Autodesk Fusion 360 part; units mm, degrees
sketch "Sketch Metalens Holder" plane through (0, 0, 0) normal (1, 0, 0) x (0, 0, -1)
  line L0 (0, 8.15) -> (16.5, 8.15)
  line L1 (16.5, 8.15) -> (16.5, -8.35)
  line L2 (16.5, -8.35) -> (0, -8.35)
  line L3 (0, -8.35) -> (0, 8.15)
  dimension "d3" = 16.5
  dimension "d4" = 16.5
extrude "Extrude Metalens Holder" add sketch "Sketch Metalens Holder" along normal blind 6
shell "Shell Metalens Holder" thickness 1.1 removed faces 2 at (6, 2.65, -5.5) at (0, 2.65, -5.5)
sketch "Sketch Screwing Parts" plane through (0, 0, 0) normal (1, 0, 0) x (0, 0, -1)
  line L0 (0, -8.35) -> (16.5, -8.35)
  line L1 (3.5, 8.15) -> (18, 8.15)
  line L2 (18, 8.15) -> (18, 35.85)
  line L3 (18, 35.85) -> (3.5, 35.85)
  line L4 (3.5, 35.85) -> (3.5, 8.15)
  line L5 (3.5, -8.35) -> (18, -8.35)
  line L6 (18, -8.35) -> (18, -36.05)
  line L7 (18, -36.05) -> (3.5, -36.05)
  line L8 (3.5, -36.05) -> (3.5, -8.35)
  line L9 (16.5, -8.35) -> (16.5, 8.15)
  point P0 (0, 8.15)
  dimension "d144" = 3.5
  dimension "d145" = 27.7
  dimension "d148" = 27.7
  dimension "d163" = 1.5
  dimension "d164" = 3.5
extrude "Extrude31" add sketch "Sketch Screwing Parts" along normal blind 6
ref_plane "WorkPlane1" through (3, -0.1, -8.25) normal (-1, 0, 0) x (0, 0, 1)
sketch "Sketch Inside Slit" plane through (3, 0, 0) normal (-1, 0, 0) x (0, 0, 1)
  line L0 (-15.4, 7.05) -> (-15.4, -7.25)
  line L1 (-16, 7.65) -> (-0.5, 7.65)
  line L2 (-0.5, 7.65) -> (-0.5, -7.85)
  line L3 (-0.5, -7.85) -> (-16, -7.85)
  line L4 (-16, -7.85) -> (-16, 7.65)
  line L5 (-15.4, 7.05) -> (-1.1, 7.05)
  line L6 (-1.1, 7.05) -> (-1.1, -7.25)
  line L7 (-1.1, -7.25) -> (-15.4, -7.25)
  line L8 (-15.4, -7.25) -> (-15.4, 7.05)
  line L9 (-15.4, 7.05) -> (-16, 7.05)
  line L10 (-1.1, 7.05) -> (-0.5, 7.05)
  line L11 (-1.1, -7.25) -> (-0.5, -7.25)
  line L12 (-15.4, -7.25) -> (-16, -7.25)
  point P0 (-1.1, -7.25)
  point P1 (-1.1, 7.05)
  dimension "d91" = 15.5
extrude "Extrude Inside Slit" cut sketch "Sketch Inside Slit" along normal mid plane 1 contours L2 L6 L10 L11
extrude "Extrude Inside Slit Bis" cut sketch "Sketch Inside Slit" along normal mid plane 1 contours L1 L2 L4 L5 L9 L10
extrude "Extrude Inside Slit BisBis" cut sketch "Sketch Inside Slit" along normal mid plane 1 contours L0 L4 L8 L9 L12
extrude "Extrude Inside Slit BisBisBis" cut sketch "Sketch Inside Slit" along normal mid plane 1
extrude "Extrude" cut 1 faces at (0.8333, 2.2833, -15.4) along direction (0, 0, -1) blind 1.1
extrude "Extrude22" cut 1 faces at (4.3333, 2.2833, -15.4) along direction (0, 0, -1) blind 1.1
extrude "Extrude23" cut 1 faces at (2.8333, -2.4833, -16) along direction (0, 0, -1) blind 0.5
extrude "Extrude24" add 1 faces at (2, -2.85, 0) along direction (0, 0, 1) blind 0.9
extrude "Extrude25" add 2 faces at (2, 8.15, -2.0333) (2, 8.15, -2.0333) along direction (0, 1, 0) blind 0.9
extrude "Extrude26" add 2 faces at (2, -8.35, -2.0333) (2, -8.35, -2.0333) along direction (0, -1, 0) blind 0.9
extrude "Extrude27" add 1 faces at (6, 26.9167, -8.3333) along direction (1, 0, 0) blind 4.5
extrude "Extrude28" add 1 faces at (0, 26.9167, -8.3333) along direction (-1, 0, 0) blind 4.5
extrude "Extrude29" add 1 faces at (-2.1667, 7.6167, -16.5) along direction (0, 0, -1) blind 1.5
extrude "Extrude30" add 1 faces at (-2.1667, -7.8167, -16.5) along direction (0, 0, -1) blind 1.5
sketch "Sketch11" plane through (0, 0, -18) normal (0, 0, -1) x (-1, 0, 0)
  line L0 (4.5, 35.85) -> (-10.5, 35.85)
  line L1 (-10.5, 35.85) -> (-10.5, 7.05)
  line L2 (-10.5, 7.05) -> (-3.5, 7.05)
  line L3 (-3.5, 7.05) -> (-3.5, 7.65)
  line L4 (-3.5, 7.65) -> (-2.5, 7.65)
  line L5 (-2.5, 7.65) -> (-2.5, 7.05)
  line L6 (4.5, 7.05) -> (4.5, 35.85)
  circle A0 centre (-3, 30.3) radius 3.75
  line L7 (-2.5, 7.05) -> (4.5, 7.05)
  dimension "d154" = 7.5
extrude "Extrude32" cut sketch "Sketch11" against normal blind 14.5 contours A0
sketch "Sketch12" plane through (0, 0, -18) normal (0, 0, -1) x (-1, 0, 0)
  line L0 (-10.5, -7.25) -> (-10.5, -36.05)
  line L1 (-10.5, -36.05) -> (4.5, -36.05)
  line L2 (4.5, -36.05) -> (4.5, -7.25)
  line L3 (4.5, -7.25) -> (-2.5, -7.25)
  line L4 (-2.5, -7.25) -> (-2.5, -7.85)
  line L5 (-2.5, -7.85) -> (-3.5, -7.85)
  line L6 (-3.5, -7.85) -> (-3.5, -7.25)
  line L7 (-3.5, -7.25) -> (-10.5, -7.25)
  circle A0 centre (-2.9472, -30.4996) radius 3.75
  dimension "d159" = 7.5
extrude "Extrude33" cut sketch "Sketch12" against normal blind 14.5 contours A0
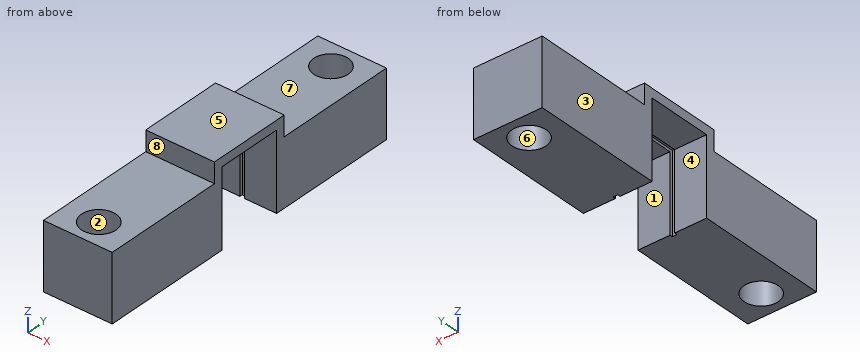
Work out the finished part from the listing and answer in its coordinate system (mm). Face numbers are marked on the shaded views. A direction names the side the tool comes from. Round coordinates to 2 decimals unless told otherwise and drop trailing zeros. Loops run counter-clockwise (first coordinate to the right, second up) from the corner with the lowest first, then second, coordinate; pieces in that order, holes last. Notation, with made-up numbers: (11, 37) - (38, 37) arc R27 ccw to (38, 73) - close; hole circle Ø4 at (59.5, 87). An arc over 180 degrees is marked (long way). Use one line per item in the form item = value. Start each with the question number.
(1) Find section A-A on z = -10.5. Determine the outline of the cut face in (x, y), and give its area (3 significant figures).
(2) Determine the mould class of the marked faces 1, 2 and 3 for opening direction X: +X half, -X half, draft (parallel to the pull), parting line (faces both ways), or undercut.
(3) Find section C-C on x = 1. Determine the outline of the cut face in (y, z), and give its area (3 significant figures).
(4) Find section B-B on y = 30.3. Determine the outline of the cut face in (x, z), and give its area (3 significant figures).
(5) Flat-ended cylindrical pins translate along their axes: P1, Ø8, axis at y = -3.5, z = -7, coming from the +X side; P2, Ø5.5, axis at x = 8, y = 1, coming from the -Z side; P3, Ø2, axis at x = 1, z = -0.5, coming from the -Y side; P4, Ø3.5, axis at x = 2, z = -0.5, coming from the +Y side. Find the tip coordinate at first contact, or state that the pin passes through.
(6) Which of the six approach directions +Z, -Z, +X, -X, +Y, -Y give full straight-line access (tool end or side, diameter ignored) to the marked faces 4, 5, 6, 7 and 8?
(7) Consider line 1 (Y direction, x = 3, z = -14.5); line 2 (Y direction, x = 1.5, z = -15.25); line 3 (Y direction, x = 4.75, z = -2.5). Determine where each line is inside the solid, lowest interval first.
(8) Find section D-D on y = 2.5. Determine the outline of the cut face in (x, z).
Answer list:
q1.outline = (-4.5, -36.05) - (10.5, -36.05) - (10.5, -7.25) - (3.5, -7.25) - (3.5, -7.85) - (2.5, -7.85) - (2.5, -7.25) - (-4.5, -7.25) - close; (-4.5, 7.05) - (2.5, 7.05) - (2.5, 7.65) - (3.5, 7.65) - (3.5, 7.05) - (10.5, 7.05) - (10.5, 35.85) - (-4.5, 35.85) - close; hole circle Ø7.5 at (2.95, -30.5); hole circle Ø7.5 at (3, 30.3)
q1.area = 774 mm^2
q2.face_1 = draft
q2.face_2 = undercut
q2.face_3 = -X half
q3.outline = (-36.05, -18) - (-33.7, -18) - (-33.7, -3.5) - (-36.05, -3.5) - close; (-27.29, -18) - (-7.25, -18) - (-7.25, -1.1) - (7.05, -1.1) - (7.05, -18) - (27.13, -18) - (27.13, -3.5) - (9.05, -3.5) - (9.05, 0.9) - (-9.25, 0.9) - (-9.25, -3.5) - (-27.29, -3.5) - close; (33.47, -18) - (35.85, -18) - (35.85, -3.5) - (33.47, -3.5) - close
q3.area = 696 mm^2
q4.outline = (-4.5, -18) - (-0.75, -18) - (-0.75, -3.5) - (-4.5, -3.5) - close; (6.75, -18) - (10.5, -18) - (10.5, -3.5) - (6.75, -3.5) - close
q4.area = 109 mm^2
q5.P1 = 10.5
q5.P2 = -1.1
q5.P3 = -9.25
q5.P4 = 9.05
q6.face_4 = -Z, +X, -X
q6.face_5 = +Z, +X, -X, +Y, -Y
q6.face_6 = +Z, -Z
q6.face_7 = +Z, +X, -X, +Y
q6.face_8 = +Z, +X, -X, -Y
q7.line_1 = -36.05 to -34.25, -26.75 to -7.85, 7.65 to 26.55, 34.05 to 35.85
q7.line_2 = -36.05 to -33.96, -27.04 to -7.25, 7.05 to 26.86, 33.74 to 35.85
q7.line_3 = -9.25 to -7.25, 7.05 to 9.05
q8.outline = (-4.5, -1.1) - (2.5, -1.1) - (2.5, -0.5) - (3.5, -0.5) - (3.5, -1.1) - (10.5, -1.1) - (10.5, 0.9) - (-4.5, 0.9) - close
